Geometry: final body of the model. Coordinates: model frame, mm. Round coordinates to 2 decimals unless told otherwise and drop trailing zeros. Write each loop counter-clockwise with the first axis right and the second up, starting at its lowest first coordinate (ties: lowest second). Pieces come first, ordered by that corner, then holes. Notation, with made-up numbers: M 35,-4.75 L 48,-4.75 A34 cw 48,34.25 Z; hole C -1,-2.75 d7. An arc over 180 degrees is marked long. Put each result on its own line as item: value. Start each with the question number.
```python
from build123d import *

# Parameters (mm, degrees)
SKETCH2_R                    = 35
BOSS_EXTRUDE1_DEPTH          = 1.5875
SKETCH3_R                    = 7
CUT_EXTRUDE1_DEPTH           = 4.175
M3_CLEARANCE_HOLE1_D         = 3.4
CSK_FOR_M4_SFHCS1_AT_2_COUNT = 2
CSK_FOR_M4_SFHCS1_AT_2_PITCH = 10
CSK_FOR_M4_SFHCS1_AT_3_COUNT = 2
CSK_FOR_M4_SFHCS1_AT_3_PITCH = 45
CSK_FOR_M4_SFHCS1_AT_4_COUNT = 2
CSK_FOR_M4_SFHCS1_AT_4_PITCH = 55


with BuildPart() as part:
    # Sketch2 → Boss-Extrude1 (new body, symmetric)
    with BuildSketch(Plane.XY):
        Circle(SKETCH2_R)
    extrude(amount=BOSS_EXTRUDE1_DEPTH, both=True)

    # Sketch3 → Cut-Extrude1 (cut, through all)
    with BuildSketch(Plane.XY.offset(1.5875)):
        Circle(SKETCH3_R)
    extrude(amount=-CUT_EXTRUDE1_DEPTH, mode=Mode.SUBTRACT)

    # M3 Clearance Hole1 (through all)
    with Locations(Plane.XY.offset(1.5875)):
        with Locations((8, 5), (8, -5), (-8, 5), (-8, -5)):
            Hole(M3_CLEARANCE_HOLE1_D / 2)

    # Sketch8 → CSK for M4 SFHCS1 (revolve, cut)
    with BuildSketch(Plane(origin=(2.358e-06, 27.5, -1.5875), x_dir=(0, 1, 0), z_dir=(1, 0, 0))):
        Polygon((0, 0), (0, 3.175), (2.25, 3.175), (2.25, 2.23), (4.48, 0), align=None)
    csk_for_m4_sfhcs1 = revolve(axis=Axis((2.358e-06, 27.5, -7.9375), (0, 0, 1)), mode=Mode.SUBTRACT)

    # CSK for M4 SFHCS1 at 2: CSK for M4 SFHCS1 ×2
    with Locations(*[(0, -i * CSK_FOR_M4_SFHCS1_AT_2_PITCH, 0) for i in range(1, CSK_FOR_M4_SFHCS1_AT_2_COUNT)]):
        add(csk_for_m4_sfhcs1, mode=Mode.SUBTRACT)

    # CSK for M4 SFHCS1 at 3: CSK for M4 SFHCS1 ×2
    with Locations(*[(0, -i * CSK_FOR_M4_SFHCS1_AT_3_PITCH, 0) for i in range(1, CSK_FOR_M4_SFHCS1_AT_3_COUNT)]):
        add(csk_for_m4_sfhcs1, mode=Mode.SUBTRACT)

    # CSK for M4 SFHCS1 at 4: CSK for M4 SFHCS1 ×2
    with Locations(*[(0, -i * CSK_FOR_M4_SFHCS1_AT_4_PITCH, 0) for i in range(1, CSK_FOR_M4_SFHCS1_AT_4_COUNT)]):
        add(csk_for_m4_sfhcs1, mode=Mode.SUBTRACT)


solid = part.part
```
1) Section A-A, the plane y = 0. Output: boundary loops of the cut face in (x, z).
2) Section C-C, the plane y = -17.5. Output: boundary loops of the cut face in (x, z), and give its area (3 significant figures).
3) First-contact query: pin 1 (1.5 mm diameter, centred on x = 3, z = 0.5, fed in from +Y); pin 2 (2 mm diameter, centred on x = -8, y = -5, fed in from +Z); pin 3 (1 mm diameter, centred on x = 16.5, z = 1, fed in from -Y). Flat tips, straight axial feed; report the tip coordinate or a pass-through.
4) Section B-B, the plane x = -8. Output: boundary loops of the cut face in (y, z).
5) Draft query along X for faces 1 (the face through (-0.5, -7.3, 1.588)), 2 (the face through (6.466, -2.681, 0.022)), 3 (the face through (-28, -21, 0)). Return one class per face: +X half, -X half, draft (parallel to the pull), parting line (faces both ways), or undercut.
6) Ray query, probe 1 along Y at (x, z) = (8, -0.75); probe 2 along Y at (x, z) = (-9.5, -0.4); probe 3 along X at (y, z) = (16, 0.55). Return the intervals inside material, ascending.
7) Section D-D, the plane x = 21. Output: boundary loops of the cut face in (y, z), and give its area (3 significant figures).
Solved:
1. outline: M -35,-1.59 L -7,-1.59 L -7,1.59 L -35,1.59 Z; M 7,-1.59 L 35,-1.59 L 35,1.59 L 7,1.59 Z
2. outline: M -30.31,-1.59 L -4.48,-1.59 L -2.25,0.64 L -2.25,1.59 L -30.31,1.59 Z; M 2.25,0.64 L 4.48,-1.59 L 30.31,-1.59 L 30.31,1.59 L 2.25,1.59 Z
2. area: 173 mm2
3. pin 1: stops at y = 34.93
3. pin 2: passes through
3. pin 3: stops at y = -31.13
4. outline: M -34.07,-1.59 L -6.7,-1.59 L -6.7,1.59 L -34.07,1.59 Z; M -3.3,-1.59 L 3.3,-1.59 L 3.3,1.59 L -3.3,1.59 Z; M 6.7,-1.59 L 34.07,-1.59 L 34.07,1.59 L 6.7,1.59 Z
5. face 1: draft
5. face 2: undercut
5. face 3: parting line
6. probe 1: y = -34.07 to -6.7, -3.3 to 3.3, 6.7 to 34.07
6. probe 2: y = -33.69 to -5.8, -4.2 to 4.2, 5.8 to 33.69
6. probe 3: x = -31.13 to -1.8, 1.8 to 31.13
7. outline: M -28,-1.59 L 28,-1.59 L 28,1.59 L -28,1.59 Z
7. area: 178 mm2
